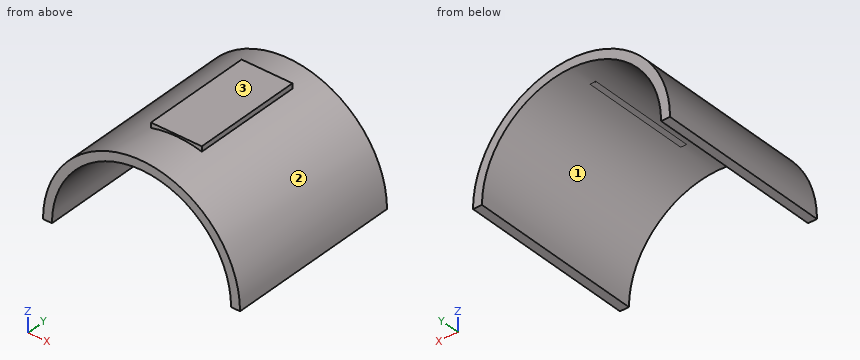
from build123d import *

# Parameters (mm, degrees)
F1_DEPTH = 30
F4_W     = 8.514822
F4_H     = 18.499203
F5_DEPTH = 1
F6_W     = 8.514822
F6_H     = 18.499203
F7_DEPTH = 1.8


with BuildPart() as f1:
    # F0 (on Front) → F1 (new body)
    with BuildSketch(Plane.XZ):
        with BuildLine():
            ThreePointArc((-15, 0), (0, 15), (15, 0))
            Line((15, 0), (16.5, 0))
            ThreePointArc((16.5, 0), (0, 16.5), (-16.5, 0))
            Line((-16.5, 0), (-15, 0))
        make_face()
    extrude(amount=F1_DEPTH)



with BuildPart() as f5:
    # F4 (on face) → F5 (new body)
    with BuildSketch(Plane.XY.offset(15.791785)):
        with Locations((0, -13.633903)):
            Rectangle(F4_W, F4_H)
    extrude(amount=F5_DEPTH)


with BuildPart() as f1_1:
    add(f1.part)

    add(f5.part)  # F7 merges F5
    # F6 (on face) → F7 (join)
    with BuildSketch(Plane.XY.offset(16.791785)):
        with Locations((0, -13.633903)):
            Rectangle(F6_W, F6_H)
    extrude(amount=-F7_DEPTH)


solid = f1_1.part
Read the model definition and answer for the solid it produces. Units are mm, in the model's axes. Face numbers are marked on the shaded views. Coordinates: 2 decimals unless noted, no trailing zeros. Order: outer loops, then holes, each group sorted by start corner. A loop starts at its lowest first (then second) coordinate and runs counter-clockwise, first axis right, second up. Notation, with made-up numbers: (0.5, 14) - (16.5, 14) arc R18 cw to (16.5, 20) - close; hole circle Ø2 at (6, 37). An arc over 180 degrees is marked (long way). Use one line per item in the form item = value.
(1) Straight lines are drawn through the part: L1, parallel to X at y = -14.25, z = 13.5; L2, parallel to X at y = -12.5, z = 2; L3, parallel to Z at x = 5.5, y = -9. For each, find the intervals that lie inside material, in ascending order.
Computed values:
L1 = -9.49 to -6.54, 6.54 to 9.49
L2 = -16.38 to -14.87, 14.87 to 16.38
L3 = 13.96 to 15.56
(2) Given pin 1 Ø0.9 at (y, z) = (-15.5, 16.5) entering from -X; pin 2 Ø8 at (x, z) = (8.5, 15) entering from -Y; pin 3 Ø6 at (y, z) = (-8, 10) entering from -X; pin 4 Ø1.5 at (x, z) = (10, 15) entering from -Y, each flat-ended and moving along its own axis, determine where each tip first touches the part or whether it passes through.
Computed values:
pin_1 = -4.26
pin_2 = -30
pin_3 = -14.94
pin_4 = through
(3) Section D-D, the plane z = 2.5 is taken. Give the vertices of the cut face in (x, y), then the cut area to 3 significant figures.
Computed values:
outline = (-16.31, -30) - (-14.79, -30) - (-14.79, 0) - (-16.31, 0) - close; (14.79, -30) - (16.31, -30) - (16.31, 0) - (14.79, 0) - close
area = 91.2 mm²
(4) Section C-C, the plane y = -1.75 is taken. Give the vertices of the cut face in (x, z).
Computed values:
outline = (-16.5, 0) - (-15, 0) arc R15 cw to (15, 0) - (16.5, 0) arc R16.5 ccw to start
(5) For a pull along X with two mould halves and no side action, classify the marked faces 1, 2 and 3 as pulls with the +X half, pulls with the -X half, needs draft (parallel to the pull), parting line crosses it, or undercut.
Computed values:
face_1 = undercut
face_2 = parting line crosses it
face_3 = needs draft
(6) Section A-A, the plane z = 7.25 is taken. Give the vertices of the cut face in (x, y), then the cut area to 3 significant figures.
Computed values:
outline = (-14.82, -30) - (-13.13, -30) - (-13.13, 0) - (-14.82, 0) - close; (13.13, -30) - (14.82, -30) - (14.82, 0) - (13.13, 0) - close
area = 101 mm²
